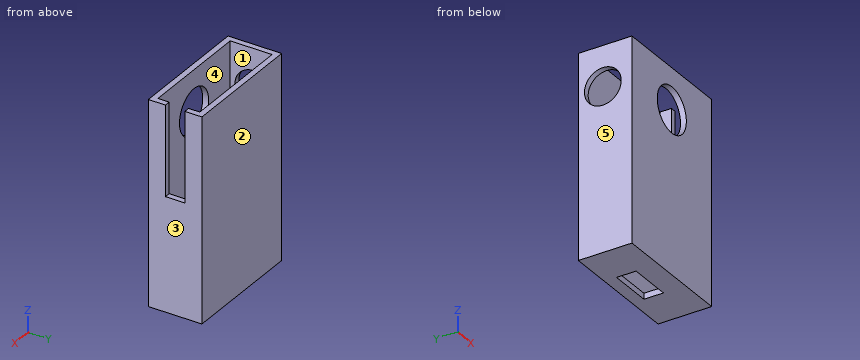
from build123d import *

# Parameters (mm, degrees)
F0_W      = 32
F0_H      = 52
F1_DEPTH  = 13.75
F2_T      = -1.5
F3_R      = 5.84
F4_DEPTH  = 1.5
F5_R      = 4.722056
F6_DEPTH  = 3
F7_W      = 5
F7_H      = 23
F8_DEPTH  = 2
F9_W      = 11
F9_H      = 5
F10_DEPTH = 2


with BuildPart() as f1:
    # F0 (on Front) → F1 (new body)
    with BuildSketch(Plane.XZ):
        Rectangle(F0_W, F0_H)
    extrude(amount=-F1_DEPTH)

    # F2
    f2_openings = [f1.faces().sort_by_distance(p)[0] for p in [
        (0, 6.875, 26),
    ]]
    offset(amount=F2_T, openings=f2_openings)

    # F3 (on Front) → F4 (cut)
    with BuildSketch(Plane.XZ):
        with Locations((0, 15.42)):
            Circle(F3_R)
    extrude(amount=-F4_DEPTH, mode=Mode.SUBTRACT)

    # F5 (on face) → F6 (cut)
    with BuildSketch(Plane(origin=(-16, 0, 0), x_dir=(0, -1, 0), z_dir=(-1, 0, 0))):
        with Locations((-7.457727, 15.722008)):
            Circle(F5_R)
    extrude(amount=-F6_DEPTH, mode=Mode.SUBTRACT)

    # F7 (on face) → F8 (cut)
    with BuildSketch(Plane.YZ.offset(16)):
        with Locations((6.88, 14.5)):
            Rectangle(F7_W, F7_H)
    extrude(amount=-F8_DEPTH, mode=Mode.SUBTRACT)

    # F9 (on face) → F10 (cut)
    with BuildSketch(Plane(origin=(0, 0, -26), x_dir=(1, 0, 0), z_dir=(0, 0, -1))):
        with Locations((0, -8.16)):
            Rectangle(F9_W, F9_H)
    extrude(amount=-F10_DEPTH, mode=Mode.SUBTRACT)


solid = f1.part
Can you work these out from the model? Positions are in its coordinate system, mm. Face numbers are marked on the shaded views. A direction names the side the tool comes from. Give positions to 0.01 mm unless a question says otherwise; leave off trailing zeros. Order: outer loops, then holes, each group sorted by start corner. A loop starts at its lowest first (then second) coordinate and runs counter-clockwise, first axis right, second up. Notation, with made-up numbers: M 32,52.5 L 63,52.5 A20 ccw 63,91.5 Z; hole C 77,64 d6. An arc over 180 degrees is marked long. Use a Markdown table: item, result. Add a question column.
Item 1: Suppose I cut it at A-A (z = -17.5). List the corners of the cut face in (x, y) for me.
Item 2: If I drill on L1, parallel to Y at x = 4.5, z = 8.5; L2, parallel to X at y = 10.5, z = -22; L3, parallel to Z at x = 0, y = 0.45, over which ranges is the centre line in solid material (lowest first)? Write a range as [from, to].
Item 3: Suppose I cut it at D-D (x = -10.5). List the corners of the cut face in (y, z) for me, then the cut area to 3 significant figures.
Item 4: For the marked faces 4 and 5, which set-ups out of +Z, -Z, +X, -X, +Y, -Y let a thin tool reach every point of the face, with its end or its side?
Item 5: Suppose I cut it at C-C (y = 3.5). List the corners of the cut face in (x, z) for me.
Item 6: Suppose I cut it at B-B (x = 0). List the corners of the cut face in (y, z) for me.
Item 7: Will these pins go through, and if not, where does the flat tip stop? pin 1 (0.8 mm diameter, centred on x = 15, y = 6, fed in from +Z); pin 2 (1.5 mm diameter, centred on x = -10.5, y = 7, fed in from +Z); pin 3 (9.5 mm diameter, centred on x = 0, z = 15.42, fed in from -Y).
Item 8: We'd pull the mould along X, two halves only. Please class the marked faces 1, 2 and 3: +X half, -X half, draft (parallel to the pull), parting line (faces both ways), or undercut.
Answer sheet:
| question | item | result |
|---|---|---|
| 1 | outline | M -16,0 L 16,0 L 16,13.75 L -16,13.75 Z; hole M -14.5,1.5 L 14.5,1.5 L 14.5,12.25 L -14.5,12.25 Z |
| 2 | L1 | y = [0, 1.5], [12.25, 13.75] |
| 2 | L2 | x = [-16, -14.5], [14.5, 16] |
| 2 | L3 | z = [-26, 9.58], [21.26, 26] |
| 3 | outline | M 0,-26 L 13.75,-26 L 13.75,26 L 12.25,26 L 12.25,-24.5 L 1.5,-24.5 L 1.5,26 L 0,26 Z |
| 3 | area | 172 mm² |
| 4 | face 4 | +Z |
| 4 | face 5 | +Z, -Z, -X, +Y, -Y |
| 5 | outline | M -16,-26 L 16,-26 L 16,26 L 14.5,26 L 14.5,-24.5 L -14.5,-24.5 L -14.5,13.15 L -16,13.15 Z; M -16,18.3 L -14.5,18.3 L -14.5,26 L -16,26 Z |
| 6 | outline | M 0,-26 L 5.66,-26 L 5.66,-24.5 L 1.5,-24.5 L 1.5,9.58 L 0,9.58 Z; M 0,21.26 L 1.5,21.26 L 1.5,26 L 0,26 Z; M 10.66,-26 L 13.75,-26 L 13.75,26 L 12.25,26 L 12.25,-24.5 L 10.66,-24.5 Z |
| 7 | pin 1 | stops at z = 3 |
| 7 | pin 2 | stops at z = -24.5 |
| 7 | pin 3 | stops at y = 12.25 |
| 8 | face 1 | undercut |
| 8 | face 2 | draft |
| 8 | face 3 | +X half |
